For this review, take the finished solid that the model builds, in its own axes (mm). Coordinates: 2 decimals unless noted, no trailing zeros. Order: outer loops, then holes, each group sorted by start corner. A loop starts at its lowest first (then second) coordinate and runs counter-clockwise, first axis right, second up. Notation, with made-up numbers: M -16.5,10 L 14.5,10 A22 cw 14.5,31 Z; hole C 77,65 d3. An arc over 180 degrees is marked long. Use CSV: the item, a comma, the result in double quotes.
```python
from build123d import *

# Parameters (mm, degrees)
F3_DEPTH      = 61.9125
F5_DEPTH      = 50.8
F5_DEPTH_BACK = 3.175
F7_DEPTH      = 1294.60625


with BuildPart() as f3:
    # F2 (on offset) → F3 (new body)
    with BuildSketch(Plane.XZ.offset(-3.175)):
        Polygon((0, 2454.275), (0, 0), (19.05, 0), (31.75, 0), (31.75, 2441.575), (311.15, 2441.575), (311.15, 0), (323.85, 0), (342.9, 0), (361.95, 0), (374.65, 0), (374.65, 2441.575), (1262.85625, 2441.575), (1262.85625, 0), (1275.55625, 0), (1294.60625, 0), (1294.60625, 2454.275), (1294.60625, 2473.325), (0, 2473.325), align=None)
    extrude(amount=-F3_DEPTH)

    # F4 (on Front) → F5 (join, two sides)
    with BuildSketch(Plane.XZ) as f5_sk:
        Polygon((0, 2454.275), (0, 0), (19.05, 0), (19.05, 2441.575), (19.05, 2454.275), (323.85, 2454.275), (323.85, 0), (342.9, 0), (361.95, 0), (361.95, 2454.275), (1275.55625, 2454.275), (1275.55625, 2441.575), (1275.55625, 0), (1294.60625, 0), (1294.60625, 2454.275), (1294.60625, 2473.325), (0, 2473.325), align=None)
    extrude(amount=F5_DEPTH)
    extrude(f5_sk.sketch, amount=-F5_DEPTH_BACK)

    # F6 (on Right) → F7 (join, through all)
    with BuildSketch(Plane.YZ):
        Polygon((32.54375, 12.7), (-18.25625, 12.7), (-56.35625, 0), (-50.8, 0), (7.14375, 0), (65.0875, 0), (70.64375, 0), align=None)
    extrude(amount=F7_DEPTH)


solid = f3.part
```
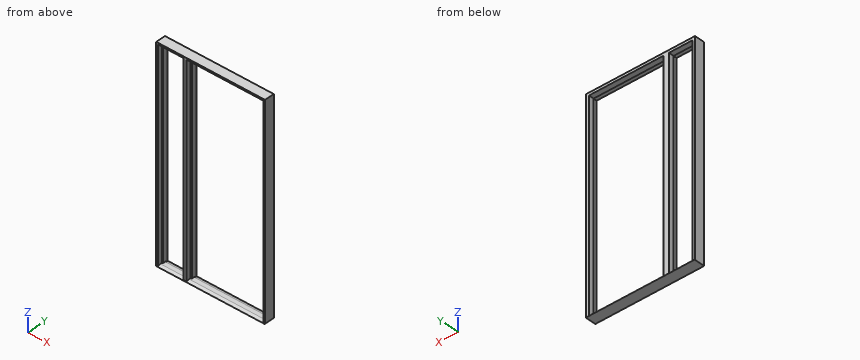
Item 1: Add section B-B on z = 919. State how many separate pieces and enclosed holes the cut face has, and give its area (3 significant figures).
Solutions:
separate pieces,"3"
enclosed holes,"0"
area,"12,000 mm^2"
Item 2: Add section A-A on x = 258. State the section outline as (y, z) points (1 decimal), and give its area (3 significant figures).
Solutions:
outline,"M -56.4,0 L 70.6,0 L 32.5,12.7 L -18.3,12.7 Z; M -50.8,2454.3 L 3.2,2454.3 L 3.2,2441.6 L 65.1,2441.6 L 65.1,2473.3 L -50.8,2473.3 Z"
area,"4,120 mm^2"
Item 3: To check wall thickness, follow line 1 along X through (y, z) = (-18, 1641); line 2 along X through (y, z) = (42, 1392); line 3 along Z through (x, y) = (779, 28.5) (3 decimals). State the ranges of each line that lie inside material, in increasing order. Write a range as [from, to].
Solutions:
line 1,"[0, 19.05], [323.85, 361.95], [1275.56, 1294.61]"
line 2,"[0, 31.75], [311.15, 374.65], [1262.86, 1294.61]"
line 3,"[0, 12.7], [2441.575, 2473.325]"
